Check sheet for the modelled part. Datum: model origin and axes. Units: mm. Give positions to 0.01 mm unless a question says otherwise; leave off trailing zeros. Write each loop counter-clockwise with the first axis right and the second up, starting at its lowest first coordinate (ties: lowest second). Pieces come first, ordered by that corner, then holes. Notation, with made-up numbers: (0, -9) -> (45, -9) arc R20 ccw to (45, 7) -> close; hole circle Ø1 at (-3.75, 44.25). An arc over 180 degrees is marked (long way). Use a Markdown table: item, result. Add a question column.
1. Release check for a two-part mould opening along Z. For faces 1 (the flat face through (2, 0, 140)), 2 (the flat face through (1.972, 15.207, 68.772)), 3 (the cylindrical face through (2.028, 1.201, 124.343)) record: released by +Z, released by -Z, zero draft, split by the parting line, or undercut.
2. Cross-section at A-A (x = 1.25). Enter the section's corners in (y, z).
3. Cross-section at B-B (z = 87). Enter the section's corners in (x, y).
4. Scan lines: probe 1 along Y at (x, z) = (2.2, 0); probe 2 along Z at (x, y) = (1.75, 2.5); probe 3 along Y at (x, z) = (1.05, 7.24). Record each from-to range of solid material in increasing order. Write a range as [from, to].
5. Cross-section at C-C (z = 27). Enter the section's corners in (x, y).
from build123d import *

# Parameters (mm, degrees)
SKETCH1_R           = 4
SKETCH1_R_2         = 0.7
BOSS_EXTRUDE1_DEPTH = 4
SKETCH2_R           = 4
CUT_EXTRUDE1_DEPTH  = 10


with BuildPart() as part:
    # Sketch1 → Boss-Extrude1 (new body)
    with BuildSketch(Plane(origin=(0, 0, 0), x_dir=(0, 0, -1), z_dir=(1, 0, 0))):
        with BuildLine():
            Line((-140, 18), (-140, -18))
            Line((-140, -18), (0.489836976, -12.490398702))
            ThreePointArc((0.489836976, -12.490398702), (12.5, 0), (0.489836976, 12.490398702))
            Line((0.489836976, 12.490398702), (-140, 18))
        make_face()
        Circle(SKETCH1_R, mode=Mode.SUBTRACT)
        with Locations((-7.24, 0)):
            Circle(SKETCH1_R_2, mode=Mode.SUBTRACT)
        with Locations((0, 7.24)):
            Circle(SKETCH1_R_2, mode=Mode.SUBTRACT)
        with Locations((7.24, 0)):
            Circle(SKETCH1_R_2, mode=Mode.SUBTRACT)
        with Locations((0, -7.24)):
            Circle(SKETCH1_R_2, mode=Mode.SUBTRACT)
    extrude(amount=BOSS_EXTRUDE1_DEPTH)

    # Sketch2 → Cut-Extrude1 (cut)
    with BuildSketch(Plane(origin=(4, 0, 0), x_dir=(0, 0, -1), z_dir=(1, 0, 0))):
        with Locations((-128.15876547, 0)):
            Circle(SKETCH2_R)
    extrude(amount=-CUT_EXTRUDE1_DEPTH, mode=Mode.SUBTRACT)


solid = part.part
Worked answers:
| question | item | result |
|---|---|---|
| 1 | face 1 | released by +Z |
| 1 | face 2 | released by -Z |
| 1 | face 3 | undercut |
| 2 | outline | (-18, 140) -> (-12.49, -0.49) arc R12.5 ccw to (12.49, -0.49) -> (18, 140) -> close; hole circle Ø1.4 at (-7.24, 0); hole circle Ø8 at (0, 0); hole circle Ø8 at (0, 128.16); hole circle Ø1.4 at (0, -7.24); hole circle Ø1.4 at (0, 7.24); hole circle Ø1.4 at (7.24, 0) |
| 3 | outline | (0, -15.92) -> (4, -15.92) -> (4, 15.92) -> (0, 15.92) -> close |
| 4 | probe 1 | y = [-12.51, -7.94], [-6.54, -4], [4, 6.54], [7.94, 12.51] |
| 4 | probe 2 | z = [-12.25, -3.12], [3.12, 125.04], [131.28, 140] |
| 4 | probe 3 | y = [-12.79, -0.7], [0.7, 12.79] |
| 5 | outline | (0, -13.57) -> (4, -13.57) -> (4, 13.57) -> (0, 13.57) -> close |
